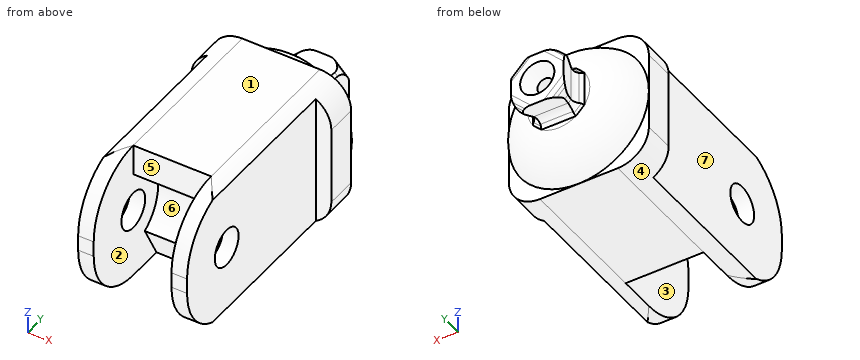
from build123d import *

# Parameters (mm, degrees)
SKETCH4_W           = 17
SKETCH4_H           = 11
BOSS_EXTRUDE2_DEPTH = 8.5
CUT_EXTRUDE1_DEPTH  = 13.5
CUT_EXTRUDE2_DEPTH  = 13.5
CUT_EXTRUDE3_DEPTH  = 13.5
CUT_EXTRUDE4_DEPTH  = 13.5
FILLET1_R           = 2
SKETCH16_W          = 45
SKETCH16_H          = 45
BOSS_EXTRUDE3_DEPTH = 75
SKETCH17_W          = 5
SKETCH17_H          = 65
CUT_EXTRUDE5_DEPTH  = 104.544676
SKETCH18_R          = 6
CUT_EXTRUDE6_DEPTH  = 102.471671
CUT_EXTRUDE7_DEPTH  = 12.5
SKETCH20_R          = 1.5
CUT_EXTRUDE8_DEPTH  = 75
FILLET2_R           = 20
FILLET3_START       = -90.5
FILLET3_DEPTH       = 75


with BuildPart() as part:
    # Sketch4 → Boss-Extrude2 (new, symmetric)
    with BuildSketch(Plane.XY):
        Rectangle(SKETCH4_W, SKETCH4_H)
    extrude(amount=BOSS_EXTRUDE2_DEPTH, both=True)

    # Sketch5 → Cut-Extrude1 (cut, symmetric)
    with BuildSketch(Plane(origin=(0, 0, 0), x_dir=(0, 0, -1), z_dir=(1, 0, 0))):
        with BuildLine():
            Line((8.5, 5.5), (6.50251, -1.291467))
            ThreePointArc((6.50251, -1.291467), (6.473627, -2.879228), (7.259286, -4.259286))
            Line((7.259286, -4.259286), (8.5, -5.5))
            Line((8.5, -5.5), (8.5, 5.5))
        make_face()
        with BuildLine():
            Line((-8.5, -5.5), (-7.259286, -4.259286))
            ThreePointArc((-7.259286, -4.259286), (-6.473627, -2.879228), (-6.50251, -1.291467))
            Line((-6.50251, -1.291467), (-8.5, 5.5))
            Line((-8.5, 5.5), (-8.5, -5.5))
        make_face()
    extrude(amount=CUT_EXTRUDE1_DEPTH, both=True, mode=Mode.SUBTRACT)

    # Sketch7 → Cut-Extrude2 (cut, symmetric)
    with BuildSketch(Plane.XY):
        with BuildLine():
            Line((8.5, 5.5), (6.502538, -1.291517))
            ThreePointArc((6.502538, -1.291517), (6.473662, -2.87927), (7.259319, -4.259319))
            Line((7.259319, -4.259319), (8.5, -5.5))
            Line((8.5, -5.5), (8.5, 5.5))
        make_face()
        with BuildLine():
            Line((-8.5, -5.5), (-7.259319, -4.259319))
            ThreePointArc((-7.259319, -4.259319), (-6.473662, -2.87927), (-6.502538, -1.291517))
            Line((-6.502538, -1.291517), (-8.5, 5.5))
            Line((-8.5, 5.5), (-8.5, -5.5))
        make_face()
    extrude(amount=CUT_EXTRUDE2_DEPTH, both=True, mode=Mode.SUBTRACT)

    # Sketch11 → Cut-Extrude3 (cut, symmetric)
    with BuildSketch(Plane(origin=(0, 0, 0), x_dir=(0.7071067811865509, 0, -0.7071067811865441), z_dir=(0.7071067811865441, 0, 0.7071067811865509))):
        with BuildLine():
            Line((10, -5.5), (9.159523, -4.659523))
            ThreePointArc((9.159523, -4.659523), (8.341069, -3.136307), (8.499292, -1.414383))
            Line((8.499292, -1.414383), (9.693463, 1.541294))
            ThreePointArc((9.693463, 1.541294), (9.908908, 2.799329), (9.581873, 4.033069))
            ThreePointArc((9.581873, 4.033069), (9.013209, 4.854851), (8.25, 5.5))
            Line((8.25, 5.5), (14, 5.5))
            Line((14, 5.5), (14, -5.5))
            Line((14, -5.5), (10, -5.5))
        make_face()
        with BuildLine():
            Line((-14, 5.5), (-8.25, 5.5))
            ThreePointArc((-8.25, 5.5), (-9.013209, 4.854851), (-9.581873, 4.033069))
            ThreePointArc((-9.581873, 4.033069), (-9.908908, 2.799329), (-9.693463, 1.541294))
            Line((-9.693463, 1.541294), (-8.499292, -1.414383))
            ThreePointArc((-8.499292, -1.414383), (-8.341069, -3.136307), (-9.159523, -4.659523))
            Line((-9.159523, -4.659523), (-10, -5.5))
            Line((-10, -5.5), (-14, -5.5))
            Line((-14, -5.5), (-14, 5.5))
        make_face()
    extrude(amount=CUT_EXTRUDE3_DEPTH, both=True, mode=Mode.SUBTRACT)

    # Sketch12 → Cut-Extrude4 (cut, symmetric)
    with BuildSketch(Plane(origin=(0, 0, 0), x_dir=(-0.7071067811865465, 0, -0.7071067811865486), z_dir=(0.7071067811865486, 0, -0.7071067811865465))):
        with BuildLine():
            Line((10, -5.5), (9.159523, -4.659523))
            ThreePointArc((9.159523, -4.659523), (8.341069, -3.136307), (8.499292, -1.414383))
            Line((8.499292, -1.414383), (9.693463, 1.541294))
            ThreePointArc((9.693463, 1.541294), (9.908908, 2.799329), (9.581873, 4.033069))
            ThreePointArc((9.581873, 4.033069), (9.013209, 4.854851), (8.25, 5.5))
            Line((8.25, 5.5), (14, 5.5))
            Line((14, 5.5), (14, -5.5))
            Line((14, -5.5), (10, -5.5))
        make_face()
        with BuildLine():
            Line((-14, 5.5), (-8.25, 5.5))
            ThreePointArc((-8.25, 5.5), (-9.013209, 4.854851), (-9.581873, 4.033069))
            ThreePointArc((-9.581873, 4.033069), (-9.908908, 2.799329), (-9.693463, 1.541294))
            Line((-9.693463, 1.541294), (-8.499292, -1.414383))
            ThreePointArc((-8.499292, -1.414383), (-8.341069, -3.136307), (-9.159523, -4.659523))
            Line((-9.159523, -4.659523), (-10, -5.5))
            Line((-10, -5.5), (-14, -5.5))
            Line((-14, -5.5), (-14, 5.5))
        make_face()
    extrude(amount=CUT_EXTRUDE4_DEPTH, both=True, mode=Mode.SUBTRACT)

    # Sketch14 → Cut-Revolve1 (revolve, cut)
    with BuildSketch(Plane.XY, mode=Mode.PRIVATE) as cut_revolve1_sk:
        Polygon((0, 5.5), (5.5, 5.5), (2.5, 1.5), (2.5, -5.5), (0, -5.5), align=None)
    revolve(cut_revolve1_sk.sketch.rotate(Axis((0, -5.5, 0), (0, 1, 0)), 90), axis=Axis((0, -5.5, 0), (0, 1, 0)), mode=Mode.SUBTRACT)

    # Fillet1
    fillet1_edges = [part.edges().sort_by_distance(p)[0] for p in [
        (5.833631, 5.5, -5.833631),
        (-5.833631, 5.5, -5.833631),
        (-5.833631, 5.5, 5.833631),
        (5.833631, 5.5, 5.833631),
    ]]
    fillet(fillet1_edges, radius=FILLET1_R)

    # Sketch15 → Revolve1 (revolve)
    with BuildSketch(Plane(origin=(0, 0, 0), x_dir=(0, 0, -1), z_dir=(1, 0, 0))):
        with BuildLine():
            Line((0, -15.5), (22.5, -15.5))
            ThreePointArc((22.5, -15.5), (17.455905, -8.920713), (9.998, -5.3))
            Line((9.998, -5.3), (0, -5.3))
            Line((0, -5.3), (0, -5.5))
            Line((0, -5.5), (0, -15.5))
        make_face()
    revolve(axis=Axis((0, -5.5, 0), (0, -1, 0)))

    # Sketch16 → Boss-Extrude3 (add)
    with BuildSketch(Plane.XZ.offset(15.5)):
        Rectangle(SKETCH16_W, SKETCH16_H)
    extrude(amount=BOSS_EXTRUDE3_DEPTH)

    # Sketch17 → Cut-Extrude5 (cut, through all)
    with BuildSketch(Plane.XY.offset(22.5)):
        with Locations((-20, -58)):
            Rectangle(SKETCH17_W, SKETCH17_H)
        with Locations((20, -58)):
            Rectangle(SKETCH17_W, SKETCH17_H)
    extrude(amount=-CUT_EXTRUDE5_DEPTH, mode=Mode.SUBTRACT)

    # Sketch18 → Cut-Extrude6 (cut, through all)
    with BuildSketch(Plane(origin=(17.5, 0, 0), x_dir=(0, 0, -1), z_dir=(1, 0, 0))):
        with Locations(Location((0, -70.5, 0), (0, 0, 90))):
            Circle(SKETCH18_R)
    extrude(amount=-CUT_EXTRUDE6_DEPTH, mode=Mode.SUBTRACT)

    # Sketch19 → Cut-Extrude7 (cut, symmetric)
    with BuildSketch(Plane(origin=(0, 0, 0), x_dir=(0, 0, -1), z_dir=(1, 0, 0))):
        with BuildLine():
            Line((-22.5, -90.5), (-22.5, -70.5))
            Line((-22.5, -70.5), (-12.5, -70.5))
            ThreePointArc((-12.5, -70.5), (-2.971074, -58.358224), (11.087635, -64.728142))
            Line((11.087635, -64.728142), (22.5, -58.787241))
            Line((22.5, -58.787241), (22.5, -90.5))
            Line((22.5, -90.5), (-22.5, -90.5))
        make_face()
    extrude(amount=CUT_EXTRUDE7_DEPTH, both=True, mode=Mode.SUBTRACT)

    # Sketch20 → Cut-Extrude8 (cut)
    with BuildSketch(Plane.XZ.offset(90.5)):
        with Locations(Location((-10.5, 10.5, 0), (0, 0, 270))):
            Circle(SKETCH20_R)
    extrude(amount=-CUT_EXTRUDE8_DEPTH, mode=Mode.SUBTRACT)

    # Fillet2
    fillet2_edges = [part.edges().sort_by_distance(p)[0] for p in [
        (-15, -90.5, -22.5),
        (15, -90.5, -22.5),
        (-15, -90.5, 22.5),
        (15, -90.5, 22.5),
    ]]
    fillet(fillet2_edges, radius=FILLET2_R)

    # Fillet3: read off the stored shape, not the designer's step
    # Fillet3 outline → Fillet3 (cut)
    with BuildSketch(Plane(origin=(0, 0, 0), x_dir=(1, 0, 0), z_dir=(0, 1, 0)).offset(FILLET3_START)):
        with BuildLine():
            ThreePointArc((22.5, -12.5), (19.571068, -19.571068), (12.5, -22.5))
            Line((12.5, -22.5), (22.5, -22.5))
            Line((22.5, -22.5), (22.5, -12.5))
        make_face()
        with BuildLine():
            Line((-22.5, -22.5), (-12.5, -22.5))
            ThreePointArc((-12.5, -22.5), (-19.571068, -19.571068), (-22.5, -12.5))
            Line((-22.5, -12.5), (-22.5, -22.5))
        make_face()
        with BuildLine():
            ThreePointArc((12.5, 22.5), (19.571068, 19.571068), (22.5, 12.5))
            Line((22.5, 12.5), (22.5, 22.5))
            Line((22.5, 22.5), (12.5, 22.5))
        make_face()
        with BuildLine():
            Line((-22.5, 22.5), (-22.5, 12.5))
            ThreePointArc((-22.5, 12.5), (-19.571068, 19.571068), (-12.5, 22.5))
            Line((-12.5, 22.5), (-22.5, 22.5))
        make_face()
    extrude(amount=FILLET3_DEPTH, mode=Mode.SUBTRACT)


solid = part.part
Work out the finished part from the listing and answer in its coordinate system (mm). Face numbers are marked on the shaded views. A direction names the side the tool comes from. Coordinates: 2 decimals unless noted, no trailing zeros. Write each loop counter-clockwise with the first axis right and the second up, starting at its lowest first coordinate (ties: lowest second). Pieces come first, ordered by that corner, then holes. Notation, with made-up numbers: M 57,16.5 L 108,16.5 A6 cw 108,20.5 Z; hole C 35,87 d4. An arc over 180 degrees is marked long. Answer as CSV lines item,"result". Start each with the question number.
Item 1: A tool of negligible diameter and unlimited length cuts with its end or side. For the marked faces 5, 6 and 7, from which of +Z, -Z, +X, -X, +Y, -Y can it reach the whole face along a straight path? Write none if from no direction.
Item 2: Determine the mould class of the marked faces 1, 2, 3 and 4 for opening direction Z: released by +Z, released by -Z, zero draft, split by the parting line, or undercut.
Item 3: Flat-ended cylindrical pins translate along their axes: P1, Ø1, axis at y = -38.5, z = 7, coming from the -X side; P2, Ø1.5, axis at x = -10, z = 10.5, coming from the -Y side; P3, Ø1.5, axis at x = -19, z = -4, coming from the -Y side; P4, Ø7, axis at y = -70.5, z = 0, coming from the -X side. Find the tip coordinate at first contact, or state that the pin passes through.
Item 4: Section A-A on y = -71.5 is taken. Write down the section's boundary in (x, z), and give its area (3 significant figures).
Item 5: Consider L1, parallel to X at y = -81.5, z = -18; L2, parallel to Z at x = -10.5, y = -31; L3, parallel to X at y = -56, z = 10.5. Determine where each line is inside the solid, lowest interval first.
Checks:
1,face 5,"+Z, -Z, -Y"
1,face 6,"-Y"
1,face 7,"+Z, -Z, -X, -Y"
2,face 1,"released by +Z"
2,face 2,"undercut"
2,face 3,"undercut"
2,face 4,"released by -Z"
3,P1,"stops at x = -17.5"
3,P2,"stops at y = -15.5"
3,P3,"stops at y = -25.5"
3,P4,"passes through"
4,outline,"M -17.5,-21.16 A10 ccw -13.21,-22.47 L -12.5,-22.47 L -12.5,-5.92 L -17.5,-5.92 Z; M -17.5,5.92 L -12.5,5.92 L -12.5,22.47 L -13.21,22.47 A10 ccw -17.5,21.16 Z; M 12.5,-22.47 L 13.21,-22.47 A10 ccw 17.5,-21.16 L 17.5,-5.92 L 12.5,-5.92 Z; M 12.5,5.92 L 17.5,5.92 L 17.5,21.16 A10 ccw 13.21,22.47 L 12.5,22.47 Z"
4,area,"323 mm²"
5,L1,"x = -17.5 to -12.5, 12.5 to 17.5"
5,L2,"z = -22.5 to 9, 12 to 22.5"
5,L3,"x = -17.5 to -12, -9 to 17.5"
